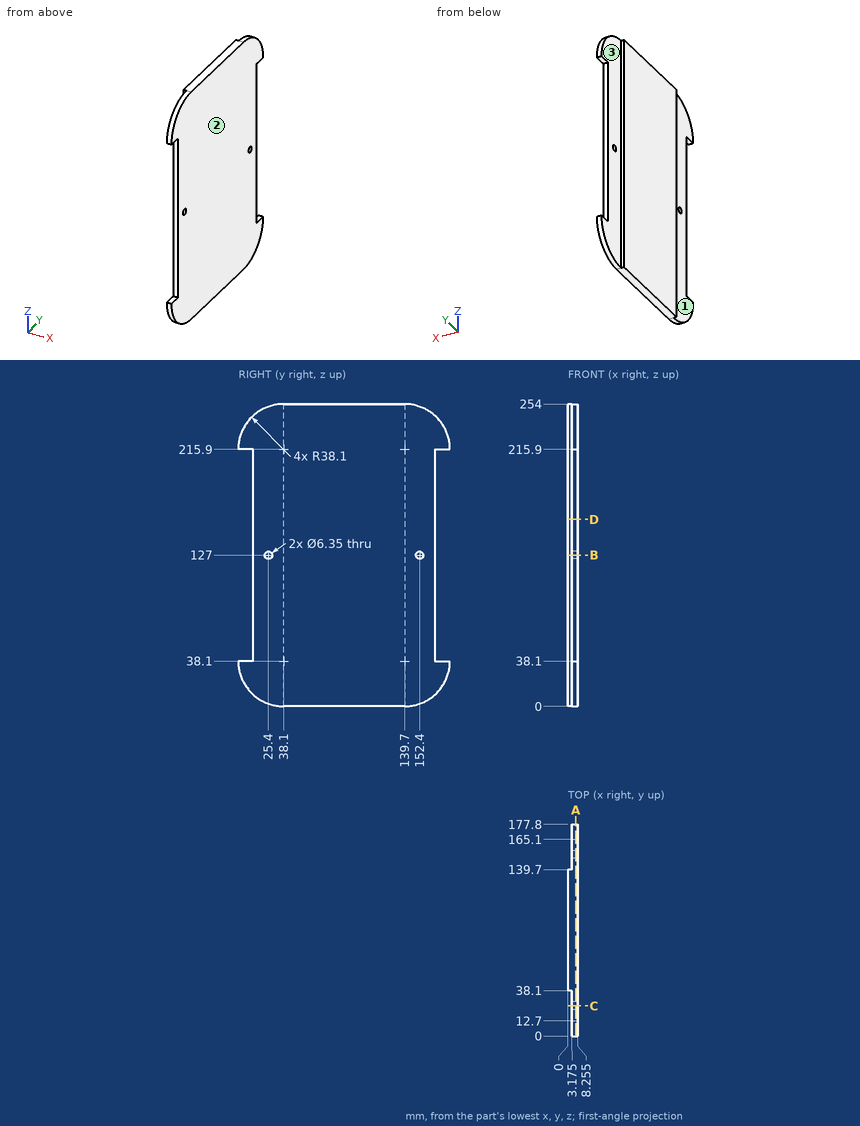
Could you check a few things on this drawing? It's one solid part, dimensions in mm from its lowest x, y, z. A direction names the side the tool comes from. Coordinates: 2 decimals unless noted, no trailing zeros. Write each loop counter-clockwise with the first axis right and the second up, starting at its lowest first coordinate (ties: lowest second). Pieces come first, ordered by that corner, then holes.
1) If we section it at C-C (y = 25.4): List the corners of the cut face in (x, z) for me (3 decimals).
Filled in:
outline: (3.175, 2.179) - (8.255, 2.179) - (8.255, 123.825) - (3.175, 123.825) - close; (3.175, 130.175) - (8.255, 130.175) - (8.255, 251.821) - (3.175, 251.821) - close
2) If I drill on line 1 (Y direction, x = 5.45, z = 127) (3 decimals); line 2 (Y direction, x = 3.75, z = 173.5); line 3 (X direction, y = 36, z = 99.5) (3 decimals), over which ranges is the centre line in solid material (lowest first)?
Filled in:
line 1: y = 12.7 to 22.225, 28.575 to 149.225, 155.575 to 165.1
line 2: y = 12.7 to 165.1
line 3: x = 3.175 to 8.255
3) If we section it at B-B (z = 127): List the corners of the cut face in (x, y) for me (3 decimals), plus the area to 3 significant figures.
Filled in:
outline: (0, 38.1) - (3.175, 38.1) - (3.175, 28.575) - (8.255, 28.575) - (8.255, 149.225) - (3.175, 149.225) - (3.175, 139.7) - (0, 139.7) - close; (3.175, 12.7) - (8.255, 12.7) - (8.255, 22.225) - (3.175, 22.225) - close; (3.175, 155.575) - (8.255, 155.575) - (8.255, 165.1) - (3.175, 165.1) - close
area: 1,030 mm2
4) Which directions (+Z, -Z, +X, -X, +Y, -Y) give clear straight access to the entire face, cutting with the end or side of a thin tool? Please do the marked faces 1, 2 and 3.
Filled in:
face 1: +Z, -Z, -X, -Y
face 2: +Z, -Z, +X, +Y, -Y
face 3: +Z, -Z, -X, +Y
5) If we section it at A-A (x = 6.75): List the corners of the cut face in (y, z) for me (3 decimals).
Filled in:
outline: (0, 38.1) arc R38.1 ccw to (38.1, 0) - (139.7, 0) arc R38.1 ccw to (177.8, 38.1) - (165.1, 38.1) - (165.1, 215.9) - (177.8, 215.9) arc R38.1 ccw to (139.7, 254) - (38.1, 254) arc R38.1 ccw to (0, 215.9) - (12.7, 215.9) - (12.7, 38.1) - close; hole circle Ø6.35 at (25.4, 127); hole circle Ø6.35 at (152.4, 127)
6) If we section it at D-D (z = 157): List the corners of the cut face in (x, y) for me (3 decimals), plus the area to 3 significant figures.
Filled in:
outline: (0, 38.1) - (3.175, 38.1) - (3.175, 12.7) - (8.255, 12.7) - (8.255, 165.1) - (3.175, 165.1) - (3.175, 139.7) - (0, 139.7) - close
area: 1,100 mm2
7) I'm going to push flat-ended pins straight in: pin 1 (8.5 mm diameter, centred on y = 152.4, z = 127, fed in from +X) (3 decimals); pin 2 (11.5 mm diameter, centred on y = 166, z = 135, fed in from -X) (3 decimals); pin 3 (3.5 mm diameter, centred on x = 2, z = 124, fed in from -Y); pin 4 (4 mm diameter, centred on x = 6, y = 7.5, fed in from -Z). Where does each tip first touch, or does it pass through?
Filled in:
pin 1: stops at x = 8.255
pin 2: stops at x = 3.175
pin 3: stops at y = 12.7
pin 4: stops at z = 12.93
